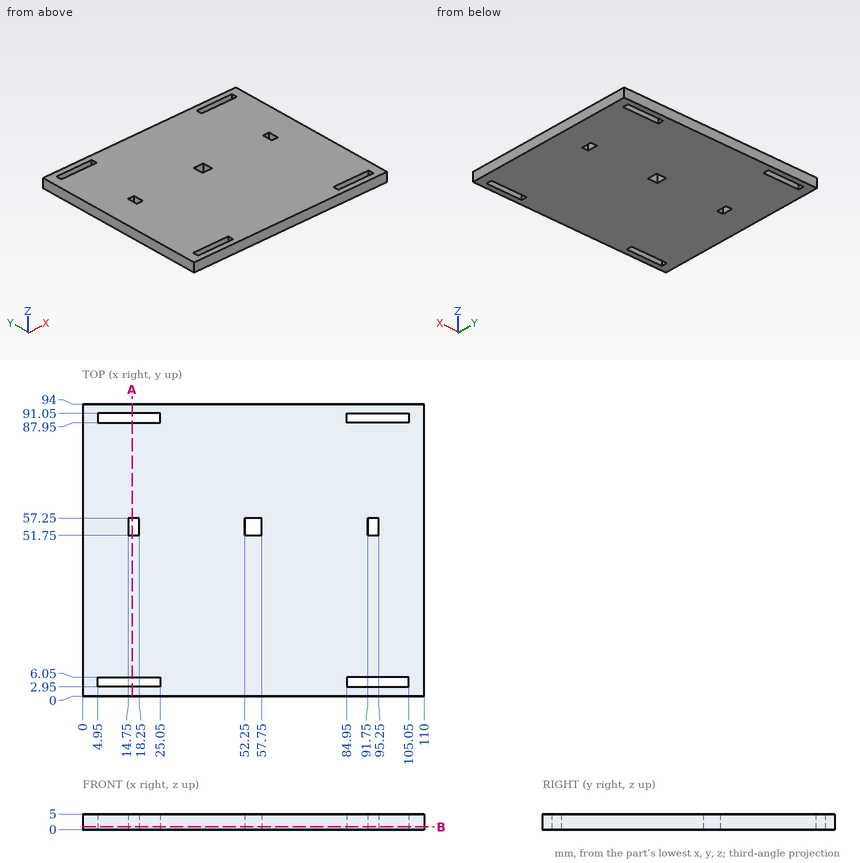
Drawing for the job (mm, zero at the part's lowest x, y, z). Coordinates: 2 decimals unless noted, no trailing zeros. Loops run counter-clockwise (first coordinate to the right, second up) from the corner with the lowest first, then second, coordinate; pieces in that order, holes last. Notation, with made-up numbers: (-5.75, -39.5) - (32.25, -39.5) arc R30 cw to (32.25, -6.5) - close; hole circle Ø7 at (38, 42.5). An arc over 180 degrees is marked (long way). Return JSON: item names as keys, results as strings.
1. Probe L1, parallel to X at y = 54, z = 2; L2, parallel to Y at x = 13, z = 3.3; L3, parallel to Y at x = 92.5, z = 1.2. List the from-to ranges inside material, lowest first. Write a range as from..to.
Result:
{"L1": "x = 0..14.75, 18.25..52.25, 57.75..91.75, 95.25..110", "L2": "y = 0..2.95, 6.05..87.95, 91.05..94", "L3": "y = 0..2.95, 6.05..51.75, 57.25..87.95, 91.05..94"}
2. Band-saw the part on A-A (x = 16). Give the cut face in (y, z).
Result:
{"outline": "(0, 0) - (2.95, 0) - (2.95, 5) - (0, 5) - close; (6.05, 0) - (51.75, 0) - (51.75, 5) - (6.05, 5) - close; (57.25, 0) - (87.95, 0) - (87.95, 5) - (57.25, 5) - close; (91.05, 0) - (94, 0) - (94, 5) - (91.05, 5) - close"}
3. Band-saw the part on B-B (z = 0.9). State how many separate pieces and enclosed holes the cut face has, and give its area (3 significant figures).
Result:
{"separate pieces": "1", "enclosed holes": "7", "area": "10,000 mm2"}
